Check sheet for the modelled part. Datum: model origin and axes. Units: mm. Face numbers are marked on the shaded views. Coordinates: 2 decimals unless noted, no trailing zeros. Write each loop counter-clockwise with the first axis right and the second up, starting at its lowest first coordinate (ties: lowest second). Pieces come first, ordered by that corner, then holes. Notation, with made-up numbers: (-18.5, 34.25) - (-2.5, 34.25) arc R17 ccw to (-2.5, 44.25) - close; hole circle Ø5 at (-24, 38). An arc over 180 degrees is marked (long way). Answer as CSV lines item,"result". Start each with the question number.
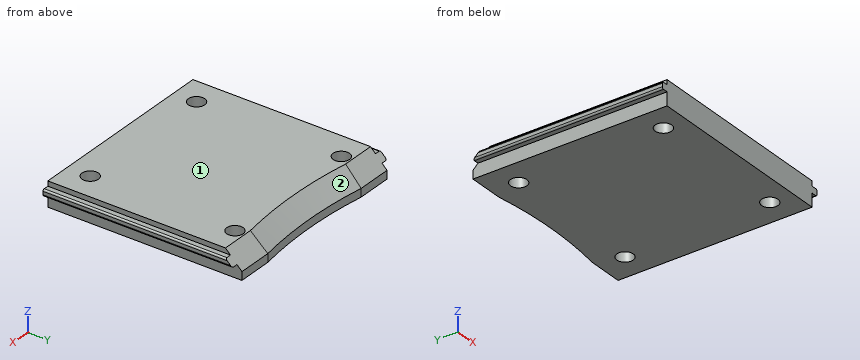
from build123d import *

# Parameters (mm, degrees)
BOSS_EXTRUDE1_DEPTH = 3.81
SKETCH3_R           = 1.27
CUT_EXTRUDE1_DEPTH  = 3.81
SKETCH4_W           = 1.016
SKETCH4_H           = 31.065921614
BOSS_EXTRUDE3_DEPTH = 1.016
FILLET2_R           = 0.254
FILLET3_R           = 0.254
SKETCH5_W           = 35.250778146
SKETCH5_H           = 1.778
CUT_EXTRUDE2_DEPTH  = 3.81
CHAMFER1_SIZE       = 2.54


with BuildPart() as part:
    # Sketch1 → Boss-Extrude1 (new body)
    with BuildSketch(Plane.XY):
        with BuildLine():
            Line((15.24, -15.875), (-15.24, -15.875))
            Line((-15.24, -15.875), (-15.24, 15.190921614))
            ThreePointArc((-15.24, 15.190921614), (0, 13.335), (15.24, 15.190921614))
            Line((15.24, 15.190921614), (15.24, -15.875))
        make_face()
    extrude(amount=BOSS_EXTRUDE1_DEPTH)

    # Sketch3 → Cut-Extrude1 (cut)
    with BuildSketch(Plane.XY.offset(3.81)):
        with Locations((-11.176, 10.033)):
            Circle(SKETCH3_R)
        with Locations((11.176, 10.033)):
            Circle(SKETCH3_R)
        with Locations((11.176, -12.319)):
            Circle(SKETCH3_R)
        with Locations((-11.176, -12.319)):
            Circle(SKETCH3_R)
    extrude(amount=-CUT_EXTRUDE1_DEPTH, mode=Mode.SUBTRACT)

    # Sketch4 → Boss-Extrude3 (add)
    with BuildSketch(Plane.ZY.offset(15.24)):
        with Locations((2.54, -0.342039193)):
            Rectangle(SKETCH4_W, SKETCH4_H)
    boss_extrude3 = extrude(amount=BOSS_EXTRUDE3_DEPTH)

    # Fillet2
    fillet2_edges = [part.edges().sort_by_distance(p)[0] for p in [
        (-16.256, -0.342039193, 2.032),
        (-16.256, -0.342039193, 3.048),
    ]]
    fillet(fillet2_edges, radius=FILLET2_R)

    # Mirror4: Boss-Extrude3 across plane
    add(boss_extrude3.mirror(Plane(origin=(0, 0, 0), x_dir=(0, 0, 1), z_dir=(1, 0, 0))))

    # Fillet3
    fillet3_edges = [part.edges().sort_by_distance(p)[0] for p in [
        (16.256, -0.342039193, 2.032),
        (16.256, -0.342039193, 3.048),
    ]]
    fillet(fillet3_edges, radius=FILLET3_R)

    # Sketch5 → Cut-Extrude2 (cut)
    with BuildSketch(Plane.XY.offset(3.81)):
        with Locations((-0.154610927, 14.986)):
            Rectangle(SKETCH5_W, SKETCH5_H)
    extrude(amount=-CUT_EXTRUDE2_DEPTH, mode=Mode.SUBTRACT)

    # Chamfer1
    chamfer1_edges = [part.edges().sort_by_distance(p)[0] for p in [
        (12.523910582, 14.097, 3.81),
        (-12.523910582, 14.097, 3.81),
        (0, 13.335, 3.81),
    ]]
    chamfer(chamfer1_edges, length=CHAMFER1_SIZE)


solid = part.part
(1) Cross-section at A-A on y = -10. Record the boundary of the cut face in (x, z).
(2) Cross-section at B-B on x = 0. Record the boundary of the cut face in (y, z) (3 decimals).
(3) Release check for a two-part mould opening along X. For the marked faces 1 and 2 record: pulls with the +X half, pulls with the -X half, needs draft (parallel to the pull), parting line crosses it, or undercut.
(4) Material ranges on probe 1 along Y at (x, z) = (10.5, 3.15) (3 decimals); probe 2 along Y at (x, z) = (-10.5, 3) (3 decimals); probe 3 along X at (y, z) = (-9.75, 1.45), recorded low to high. Write a range as from..to.
(5) Cross-section at C-C on z = 0.45. Record the boundary of the cut face in (x, y) (3 decimals).
(6) Go/stop test with flat-tipped pins: P1, Ø3, axis at x = 11.176, y = 10.033, coming from the -Z side; P2, Ø0.6, axis at y = -0.5, z = 1, coming from the +X side; P3, Ø0.8, axis at y = -4, z = 3.5, coming from the -X side. Record where each tip stops, or that it passes through.
(7) Cross-section at D-D on x = 11. Record the boundary of the cut face in (y, z) (3 decimals).
Checked values:
1,outline,"(-16.26, 2.29) arc R0.25 ccw to (-16, 2.03) - (-15.24, 2.03) - (-15.24, 0) - (15.24, 0) - (15.24, 2.03) - (16, 2.03) arc R0.25 ccw to (16.26, 2.29) - (16.26, 2.79) arc R0.25 ccw to (16, 3.05) - (15.24, 3.05) - (15.24, 3.81) - (-15.24, 3.81) - (-15.24, 3.05) - (-16, 3.05) arc R0.25 ccw to (-16.26, 2.79) - close"
2,outline,"(-15.875, 0) - (13.335, 0) - (13.335, 1.27) - (10.795, 3.81) - (-15.875, 3.81) - close"
3,face 1,"needs draft"
3,face 2,"undercut"
4,probe 1,"-15.875..-13.394, -11.244..8.958, 11.108..12.217"
4,probe 2,"-15.875..-13.394, -11.244..8.958, 11.108..12.367"
4,probe 3,"-15.24..15.24"
5,outline,"(-15.24, -15.875) - (15.24, -15.875) - (15.24, 14.097) - (9.808, 14.097) arc R63.5 cw to (-9.808, 14.097) - (-15.24, 14.097) - close; hole circle Ø2.54 at (-11.176, -12.319); hole circle Ø2.54 at (-11.176, 10.033); hole circle Ø2.54 at (11.176, -12.319); hole circle Ø2.54 at (11.176, 10.033)"
6,P1,"z = 0"
6,P2,"x = 15.24"
6,P3,"x = -15.24"
7,outline,"(-15.875, 0) - (-13.577, 0) - (-13.577, 3.81) - (-15.875, 3.81) - close; (-11.061, 0) - (8.775, 0) - (8.775, 3.81) - (-11.061, 3.81) - close; (11.291, 0) - (14.097, 0) - (14.097, 1.27) - (11.557, 3.81) - (11.291, 3.81) - close"
